```python
from build123d import *

# Parameters (mm, degrees)
F1_R     = 2
F2_DEPTH = 14
F0_R     = 40
F3_DEPTH = 5
F5_R     = 2


with BuildPart() as f2:
    # F1 (on face) → F2 (new body)
    with BuildSketch(Plane.XY):
        with Locations((0, 19.332828)):
            Circle(F1_R)
        with Locations((-20, 0)):
            Circle(F1_R)
        with Locations((20, 0)):
            Circle(F1_R)
        with Locations((0, -20)):
            Circle(F1_R)
    extrude(amount=F2_DEPTH)


with BuildPart() as f3:
    # F0 (on Top) → F3 (new body)
    with BuildSketch(Plane.XY):
        Circle(F0_R)
    extrude(amount=F3_DEPTH)

    # F4: union F2
    add(f2.part)

    # F5
    f5_edges = [f3.edges().sort_by_distance(p)[0] for p in [
        (-2, -20, 5),
        (-22, 0, 5),
        (18, 0, 5),
        (-2, 19.332828, 5),
    ]]
    fillet(f5_edges, radius=F5_R)


solid = f3.part
```
Read the model definition and answer for the solid it produces. Units are mm, in the model's axes. A direction names the side the tool comes from. Coordinates: 2 decimals unless noted, no trailing zeros. Loops run counter-clockwise (first coordinate to the right, second up) from the corner with the lowest first, then second, coordinate; pieces in that order, holes last. Notation, with made-up numbers: (46, -15.75) -> (69, -15.75) arc R9 cw to (69, -10.75) -> close; hole circle Ø9 at (11, 50.5). An arc over 180 degrees is marked (long way). Return JSON: item names as keys, results as strings.
Item 1: Find the intervals of material crossed by probe 1 along Z at (x, y) = (-28, 2.5); probe 2 along Y at (x, z) = (1, 3.5); probe 3 along Y at (x, z) = (-19, 2.25), in increasing order.
Answers:
{"probe 1": "z = 0 to 5", "probe 2": "y = -39.99 to 39.99", "probe 3": "y = -35.2 to 35.2"}
Item 2: Find section A-A (y = 0). Determine the outline of the cut face in (x, z), plus the area to 3 significant figures.
Answers:
{"outline": "(-40, 0) -> (40, 0) -> (40, 5) -> (24, 5) arc R2 cw to (22, 7) -> (22, 14) -> (18, 14) -> (18, 7) arc R2 cw to (16, 5) -> (-16, 5) arc R2 cw to (-18, 7) -> (-18, 14) -> (-22, 14) -> (-22, 7) arc R2 cw to (-24, 5) -> (-40, 5) -> close", "area": "475 mm2"}
Item 3: For a pull along Y with two mould halves and no side action, classify faces 3 (the flat face through (20, 0, 14)), 4 (the cylindrical face through (18.4, -1.2, 10.5)), 5 (the cylindrical face through (0, -18, 10)) as +Y half, -Y half, draft (parallel to the pull), parting line (faces both ways), or undercut.
Answers:
{"face 3": "draft", "face 4": "parting line", "face 5": "undercut"}
Item 4: Find section C-C (x = 20). Determine the outline of the cut face in (y, z), plus the area to 3 significant figures.
Answers:
{"outline": "(-34.64, 0) -> (34.64, 0) -> (34.64, 5) -> (4, 5) arc R2 cw to (2, 7) -> (2, 14) -> (-2, 14) -> (-2, 7) arc R2 cw to (-4, 5) -> (-34.64, 5) -> close", "area": "384 mm2"}
Item 5: For faces 1 (the flat face through (0, 19, 14)), 2 (the cylindrical face through (-0.26, 21.316, 10.451)), determine the directions among +Z, -Z, +X, -X, +Y, -Y from which every point of the face is accessible in a straight line to the end or side of a thin tool.
Answers:
{"face 1": "+Z, +X, -X, +Y, -Y", "face 2": "+Z"}
Item 6: Find section B-B (z = 6). Determine the outline of the cut face in (x, y).
Answers:
{"outline": "circle Ø4.54 at (-20, 0); circle Ø4.54 at (0, -20); circle Ø4.54 at (0, 19.33); circle Ø4.54 at (20, 0)"}
Item 7: Flat-ended cylindrical pins translate along their axes: P1, Ø4, axis at x = -29, y = 10.5, coming from the +Z side; P2, Ø24, axis at x = -4, y = -5, coming from the +Z side. Find the tip coordinate at first contact, or state that the pin passes through.
Answers:
{"P1": "stops at z = 5", "P2": "stops at z = 5.06"}
